from build123d import *

# Parameters (mm, degrees)
SKETCH1_R               = 2.25
BOSS_EXTRUDE1_DEPTH     = 40
SKETCH3_R               = 2.5
SKETCH3_W               = 15
SKETCH3_H               = 2
BOSS_EXTRUDE2_DEPTH     = 2.5
CUT_EXTRUDE2_DEPTH      = 60
CUT_EXTRUDE2_DEPTH_BACK = 60
SKETCH2_W               = 60
SKETCH2_H               = 25


with BuildPart() as part:
    # Sketch1 → Boss-Extrude1 (new, symmetric)
    with BuildSketch(Plane(origin=(0, 0, 0), x_dir=(0, 0, -1), z_dir=(1, 0, 0))):
        with BuildLine():
            Line((-20, -2.671875), (-21.75, -2.671875))
            Line((-21.75, -2.671875), (-21.75, -4.671875))
            Line((-21.75, -4.671875), (21.75, -4.671875))
            Line((21.75, -4.671875), (21.75, -2.671875))
            Line((21.75, -2.671875), (20, -2.671875))
            Line((20, -2.671875), (20, 3.328125))
            Line((20, 3.328125), (10.652726064, 3.328125))
            Line((10.652726064, 3.328125), (6, 3.328125))
            Line((6, 3.328125), (6, 9.701246493))
            Line((6, 9.701246493), (5.721159773, 11.716861618))
            ThreePointArc((5.721159773, 11.716861618), (0, 16.70104227), (-5.721159773, 11.716861618))
            Line((-5.721159773, 11.716861618), (-6, 9.701246493))
            Line((-6, 9.701246493), (-6, 3.328125))
            Line((-6, 3.328125), (-10.652726064, 3.328125))
            Line((-10.652726064, 3.328125), (-20, 3.328125))
            Line((-20, 3.328125), (-20, -2.671875))
        make_face()
        with Locations((0, 12.828125)):
            Circle(SKETCH1_R, mode=Mode.SUBTRACT)
    extrude(amount=BOSS_EXTRUDE1_DEPTH, both=True)

    # Sketch3 → Boss-Extrude2 (add)
    # profile 1 of 6: a face of its own
    with BuildSketch(Plane(origin=(0, -4.671875, 0), x_dir=(1, 0, 0), z_dir=(0, 1, 0))):
        with BuildLine():
            Line((-40, 21.75), (-48, 21.75))
            ThreePointArc((-48, 21.75), (-53, 16.75), (-48, 11.75))
            Line((-48, 11.75), (-40, 11.75))
            Line((-40, 11.75), (-40, 21.75))
        make_face()
        with Locations(Location((-48, 16.75, 0), (0, 0, 270))):
            Circle(SKETCH3_R, mode=Mode.SUBTRACT)
    # profile 2 of 6: a face of its own
    with BuildSketch(Plane(origin=(0, -4.671875, 0), x_dir=(1, 0, 0), z_dir=(0, 1, 0))):
        with BuildLine():
            Line((40, 21.75), (48, 21.75))
            ThreePointArc((48, 21.75), (53, 16.75), (48, 11.75))
            Line((48, 11.75), (40, 11.75))
            Line((40, 11.75), (40, 21.75))
        make_face()
        with Locations(Location((48, 16.75, 0), (0, 0, 90))):
            Circle(SKETCH3_R, mode=Mode.SUBTRACT)
    # profile 3 of 6: a face of its own
    with BuildSketch(Plane(origin=(0, -4.671875, 0), x_dir=(1, 0, 0), z_dir=(0, 1, 0))):
        with BuildLine():
            Line((40, -21.75), (40, -11.75))
            Line((40, -11.75), (48, -11.75))
            ThreePointArc((48, -11.75), (53, -16.75), (48, -21.75))
            Line((48, -21.75), (40, -21.75))
        make_face()
        with Locations(Location((48, -16.75, 0), (0, 0, 270))):
            Circle(SKETCH3_R, mode=Mode.SUBTRACT)
    # profile 4 of 6: a face of its own
    with BuildSketch(Plane(origin=(0, -4.671875, 0), x_dir=(1, 0, 0), z_dir=(0, 1, 0))):
        with BuildLine():
            Line((-40, -21.75), (-48, -21.75))
            ThreePointArc((-48, -21.75), (-53, -16.75), (-48, -11.75))
            Line((-48, -11.75), (-40, -11.75))
            Line((-40, -11.75), (-40, -21.75))
        make_face()
        with Locations(Location((-48, -16.75, 0), (0, 0, 90))):
            Circle(SKETCH3_R, mode=Mode.SUBTRACT)
    # profile 5 of 6: a face of its own
    with BuildSketch(Plane(origin=(0, -4.671875, 0), x_dir=(1, 0, 0), z_dir=(0, 1, 0))):
        with Locations((-47.5, 0)):
            Rectangle(SKETCH3_W, SKETCH3_H)
    # profile 6 of 6: a face of its own
    with BuildSketch(Plane(origin=(0, -4.671875, 0), x_dir=(1, 0, 0), z_dir=(0, 1, 0))):
        with Locations((47.5, 0)):
            Rectangle(SKETCH3_W, SKETCH3_H)
    extrude(amount=BOSS_EXTRUDE2_DEPTH)

    # Sketch2 → Cut-Extrude2 (cut, two sides: drawn at the far end of the back side and taken through both)
    with BuildSketch(Plane(origin=(0, -2.671875, 0), x_dir=(1, 0, 0), z_dir=(0, 1, 0)).offset(-CUT_EXTRUDE2_DEPTH_BACK)):
        Rectangle(SKETCH2_W, SKETCH2_H)
    extrude(amount=CUT_EXTRUDE2_DEPTH + CUT_EXTRUDE2_DEPTH_BACK, mode=Mode.SUBTRACT)


solid = part.part
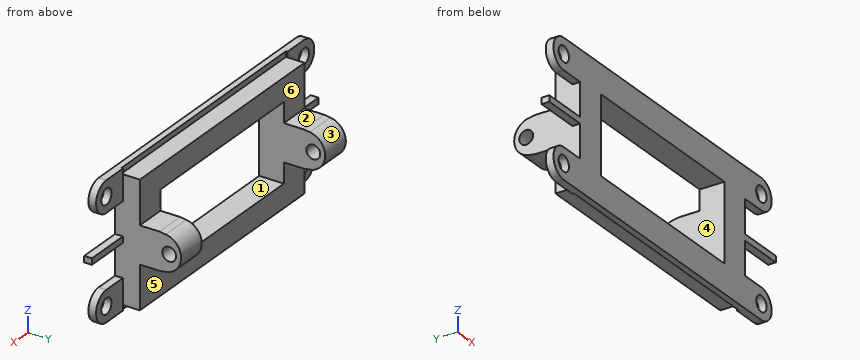
Input: part model. Units: mm. Frame: model coordinates. Face numbers are marked on the shaded views. A direction names the side the tool comes from. Coordinates: 2 decimals unless noted, no trailing zeros. Loops run counter-clockwise (first coordinate to the right, second up) from the corner with the lowest first, then second, coordinate; pieces in that order, holes last. Notation, with made-up numbers: (64, 82) -> (94, 82) arc R11 ccw to (94, 100) -> close; hole circle Ø10 at (53.5, 8). An arc over 180 degrees is marked (long way). Write item = value, one per line. Start each with the question number.
Item 1: Cut plane C-C, the plane x = -42. Return loops of the section in (y, z), plus the area to 3 significant figures.
Item 2: Cut plane D-D, the plane z = -16.75. Return loops of the section in (x, y).
Item 3: Cut plane B-B, the plane z = 0. Return loops of the section in (x, y).
Item 4: First-contact query: P1, Ø10.5, axis at y = 6.5, z = 4.5, coming from the -X side; P2, Ø8, axis at x = 46, z = -17.5, coming from the +Y side; P3, Ø8, axis at y = 14.5, z = 1.5, coming from the +X side. Flat tips, straight axial feed; report the tip coordinate or a pass-through.
Item 5: Reachability of the marked faces 4, 5 and 6 from +Z, -Z, +X, -X, +Y, -Y: full face, straight path, thin tool, end or side. Return the list, or none.
Item 6: Material intervals for line 1 (X direction, y = -2.85, z = -16.75); line 2 (Z direction, x = 9.5, y = 3.25); line 3 (X direction, y = 2, z = 7.5), sorted ascending.
Item 7: Cut plane A-A, the plane x = 13. Return loops of the section in (y, z).
Item 8: Mould query, pull axis Z, two halves, no side actions, for the marked faces 1, 2 and 3. Classes: pulls with the +Z half, pulls with the -Z half, needs draft (parallel to the pull), parting line crosses it, or undercut.
Ans:
q1.outline = (-4.67, -21.75) -> (-2.17, -21.75) -> (-2.17, -11.75) -> (-4.67, -11.75) -> close; (-4.67, -1) -> (-2.17, -1) -> (-2.17, 1) -> (-4.67, 1) -> close; (-4.67, 11.75) -> (-2.17, 11.75) -> (-2.17, 21.75) -> (-4.67, 21.75) -> close
q1.area = 55.0 mm²
q2.outline = (-53, -4.67) -> (-50.5, -4.67) -> (-50.5, -2.17) -> (-53, -2.17) -> close; (-45.5, -4.67) -> (45.5, -4.67) -> (45.5, -2.17) -> (40, -2.17) -> (40, 3.33) -> (-40, 3.33) -> (-40, -2.17) -> (-45.5, -2.17) -> close; (50.5, -4.67) -> (53, -4.67) -> (53, -2.17) -> (50.5, -2.17) -> close
q3.outline = (-55, -4.67) -> (-30, -4.67) -> (-30, 10.58) -> (-40, 10.58) -> (-40, -2.17) -> (-55, -2.17) -> close; (-40, 15.08) -> (-30, 15.08) -> (-30, 16.7) -> (-40, 16.7) -> close; (30, -4.67) -> (55, -4.67) -> (55, -2.17) -> (40, -2.17) -> (40, 10.58) -> (30, 10.58) -> close; (30, 15.08) -> (40, 15.08) -> (40, 16.7) -> (30, 16.7) -> close
q4.P1 = -40
q4.P2 = -2.17
q4.P3 = 40
q5.face_4 = +Y, -Y
q5.face_5 = -Z, +X, -X, +Y
q5.face_6 = +Z, +X, -X, +Y
q6.line_1 = -53 to -50.5, -45.5 to 45.5, 50.5 to 53
q6.line_2 = -20 to -12.5, 12.5 to 20
q6.line_3 = -40 to -30, 30 to 40
q7.outline = (-4.67, -21.75) -> (-2.67, -21.75) -> (-2.67, -20) -> (3.33, -20) -> (3.33, -12.5) -> (-4.67, -12.5) -> close; (-4.67, 12.5) -> (3.33, 12.5) -> (3.33, 20) -> (-2.67, 20) -> (-2.67, 21.75) -> (-4.67, 21.75) -> close
q8.face_1 = undercut
q8.face_2 = pulls with the +Z half
q8.face_3 = parting line crosses it
